Read the model definition and answer for the solid it produces. Units are mm, in the model's axes. A direction names the side the tool comes from. Give positions to 0.01 mm unless a question says otherwise; leave off trailing zeros. Order: outer loops, then holes, each group sorted by start corner. A loop starts at its lowest first (then second) coordinate and runs counter-clockwise, first axis right, second up.
Autodesk Inventor part; units mm, degrees
ref_plane "YZ Plane" through (0, 0, 0) normal (1, 0, 0) x (0, 1, 0)
ref_plane "XZ Plane" through (0, 0, 0) normal (0, 1, 0) x (-1, 0, 0)
ref_plane "XY Plane" through (0, 0, 0) normal (0, 0, 1) x (1, 0, 0)
sketch "Sketch1" plane through (0, 0, 0) normal (0, 0, 1) x (1, 0, 0)
  circle A0 centre (0, 0) radius 18.5
  line L0 (32, 9.5) -> (32, -22.5)
  line L1 (32, -22.5) -> (-32, -22.5)
  line L2 (-32, -22.5) -> (-32, 9.5)
  arc A1 (20.3961, 9.5) -> (-20.3961, 9.5) centre (0, 0) ccw
  line L3 (-32, 9.5) -> (-20.3961, 9.5)
  line L4 (20.3961, 9.5) -> (32, 9.5)
  point P0 (0, -22.5)
  dimension "d0" = 37
  dimension "d1" = 22.5
  dimension "d2" = 64
  dimension "d3" = 22.5
  dimension "d4" = 32
extrude "Extrusion1" add sketch "Sketch1" along normal blind 12.7
fillet "Fillet1" radius 3.175 6 edges at (32, 9.5, 6.35) (20.3961, 9.5, 6.35) (-20.3961, 9.5, 6.35) (-32, 9.5, 6.35) (-32, -22.5, 6.35) (32, -22.5, 6.35)
sketch "Sketch2" plane through (-32, -19.325, 0) normal (-1, 0, 0) x (0, 0, 1)
  line L0 (12.7, -3.175) -> (0, -3.175)
  line L1 (0, -3.175) -> (12.7, -3.175)
  point P0 (0, 19.325)
  point P1 (6.35, 20.825)
  point P2 (6.35, 4.825)
  point P3 (6.35, 0)
  dimension "d8" = 16
  dimension "d11" = 8
hole "Hole1" at (-32, 1.5, 6.35) at (-32, -14.5, 6.35) direction (1, 0, 0) diameter 2.6416 depth 11.1125 tip angle 118
sketch "Sketch4" plane through (-28.825, -22.5, 0) normal (0, -1, 0) x (1, 0, 0)
  line L0 (-3.175, 5.0292) -> (-3.175, 7.6708)
  line L1 (-3.175, 5.0292) -> (-3.175, 7.6708)
  line L2 (-3.175, 12.7) -> (-3.175, 0)
  line L3 (-3.175, 0) -> (-3.175, 12.7)
  circle A0 centre (28.825, 6.35) radius 8 construction
  point P0 (20.825, 6.35)
  point P1 (36.825, 6.35)
  point P2 (-3.175, 6.35)
  point P3 (-3.175, 6.35)
  point P4 (-3.175, 6.35)
  point P5 (4.825, 6.35)
  point P6 (52.825, 6.35)
  point P7 (-3.175, 6.35)
  dimension "d24" = 16
  dimension "d19" = 16
  dimension "d23" = 32
  dimension "d43" = 16
  dimension "d44" = 16
hole "Hole2" at (-8, -22.5, 6.35) at (8, -22.5, 6.35) at (24, -22.5, 6.35) at (-24, -22.5, 6.35) direction (0, 1, 0) diameter 2.6416 depth 11.1125 tip angle 118
mirror "Mirror1" about plane through (0, 0, 0) normal (1, 0, 0) of "Hole1"
sketch "Sketch5" plane through (0, 0, 12.7) normal (0, 0, 1) x (1, 0, 0)
  arc A0 (19.5671, 11.1076) -> (-19.5671, 11.1076) centre (0, 0) ccw
  line L0 (-28.825, -22.5) -> (28.825, -22.5)
  point P0 (-24, -6.5)
  point P1 (24, -6.5)
  dimension "d32" = 48
  dimension "d34" = 24
  dimension "d35" = 16
hole "Hole3" at (-24, -6.5, 12.7) at (24, -6.5, 12.7) direction (0, 0, -1) diameter 2.6416 end through all
properties part number "Motor Mount New - Estimated Dimensions" material "Aluminum 6061"
1) A tool of negligible diameter and unlimited length cuts with its end or side. For faces 1 (the face through (25.17, -12.58, 5.74)), 2 (the face through (31.05, -21.59, 6.44)), 3 (the face through (-26.4, 2.3, 5.3)), from which of +Z, -Z, +X, -X, +Y, -Y can it reach the whole face along a straight path? Write none if from no direction.
Final values:
face 1: -Y
face 2: +Z, -Z, +X, -Y
face 3: -X
2) Given pin 1 (4 mm diameter, centred on x = 8, z = 6.35, fed in from +Y); pin 2 (1 mm diameter, centred on x = 12, z = 9.5, fed in from +Y); pin 3 (6 mm diameter, centred on y = 10.5, z = 3.5, fed in from +X), each flat-ended and moving along its own axis, determine where each tip first touches the part or whether it passes through.
Final values:
pin 1: stops at y = 21.69
pin 2: stops at y = 19.34
pin 3: stops at x = 31.77
3) Consider L1, parallel to Y at x = -28.5, z = 6.35; L2, parallel to X at y = -12.2, z = 6.35; L3, parallel to X at y = -21, z = 6.35. Determine where each line is inside the solid, lowest interval first.
Final values:
L1: y = -22.5 to -15.82, -13.18 to 0.18, 2.82 to 9.5
L2: x = -32 to -25.32, -22.68 to -13.91, 13.91 to 22.68, 25.32 to 32
L3: x = -31.52 to -25.32, -22.68 to -9.32, -6.68 to 6.68, 9.32 to 22.68, 25.32 to 31.52
4) The part is cut by section A-A on z = 4. Determine the outline of the cut face in (x, y) (3 decimals).
Final values:
outline: (-32, -19.325) arc R3.175 ccw to (-28.825, -22.5) - (28.825, -22.5) arc R3.175 ccw to (32, -19.325) - (32, 6.325) arc R3.175 ccw to (28.825, 9.5) - (22.328, 9.5) arc R3.175 cw to (19.567, 11.108) arc R22.5 ccw to (-19.567, 11.108) arc R3.175 cw to (-22.328, 9.5) - (-28.825, 9.5) arc R3.175 ccw to (-32, 6.325) - close; hole circle Ø2.642 at (-24, -6.5); hole circle Ø37 at (0, 0); hole circle Ø2.642 at (24, -6.5)
5) The part is cut by section B-B on x = 0. Determine the outline of the cut face in (y, z).
Final values:
outline: (-22.5, 0) - (-18.5, 0) - (-18.5, 12.7) - (-22.5, 12.7) - close; (18.5, 0) - (22.5, 0) - (22.5, 12.7) - (18.5, 12.7) - close
6) The part is cut by section D-D on x = 8. Determine the outline of the cut face in (y, z).
Final values:
outline: (-22.5, 0) - (-16.68, 0) - (-16.68, 5.03) - (-22.5, 5.03) - close; (-22.5, 7.67) - (-16.68, 7.67) - (-16.68, 12.7) - (-22.5, 12.7) - close; (16.68, 0) - (21.03, 0) - (21.03, 12.7) - (16.68, 12.7) - close
7) The part is cut by section C-C on y = -2.5. Determine the outline of the cut face in (x, z), and give its area (3 significant figures).
Final values:
outline: (-32, 0) - (-18.33, 0) - (-18.33, 12.7) - (-32, 12.7) - close; (18.33, 0) - (32, 0) - (32, 12.7) - (18.33, 12.7) - close
area: 347 mm2
8) For a pull along X with two mould halves and no side action, classify faces 4 (the face through (32, -6, 6)), 5 (the face through (-22.83, -12.58, 5.74)), 6 (the face through (-0.3, 22.5, 6.3)), 7 (the face through (26.366, 2.393, 5.377)) as released by +X, released by -X, zero draft, split by the parting line, or undercut.
Final values:
face 4: released by +X
face 5: undercut
face 6: split by the parting line
face 7: zero draft
